Here's the drawing with two shaded views (mm, measured from the low corner). I have some questions. Give positions to 0.01 mm unless a question says otherwise; leave off trailing zeros. Loops run counter-clockwise (first coordinate to the right, second up) from the corner with the lowest first, then second, coordinate; pieces in that order, holes last. Notation, with made-up numbers: (-5.75, -38) - (44.25, -38) arc R29 cw to (44.25, -17) - close; hole circle Ø1 at (31.25, 16.25). An arc over 180 degrees is marked (long way). Answer as a JSON object with one key per item and string values. Group by question number.
Item 1: Suppose I cut it at B-B on z = 24. Write out the boundary of the cut face in (x, y), and give its area (3 significant figures).
Item 2: Suppose I cut it at A-A on x = 24. Write out the boundary of the cut face in (y, z), and give its area (3 significant figures).
Item 3: Suppose I cut it at C-C on y = 1.95. Write out the boundary of the cut face in (x, z), and give its area (3 significant figures).
Item 4: Thinking about a two-plate mould opening in X: for the marked faces 1 and 2, which applies, pulls with the +X half, pulls with the -X half, needs draft (parallel to the pull), parting line crosses it, or undercut?
Item 5: Will these pins go through, and if not, where does the flat tip stop? pin 1 (1.5 mm diameter, centred on x = 35, y = 0.5, fed in from -Z); pin 2 (7 mm diameter, centred on x = 20, z = 27, fed in from -Y).
Item 6: Please list where these lines run through material, in increasing order: L1, parallel to X at y = 0.3, z = 24; L2, parallel to Y at x = 39, z = 29; L3, parallel to X at y = 1.15, z = 26.5.
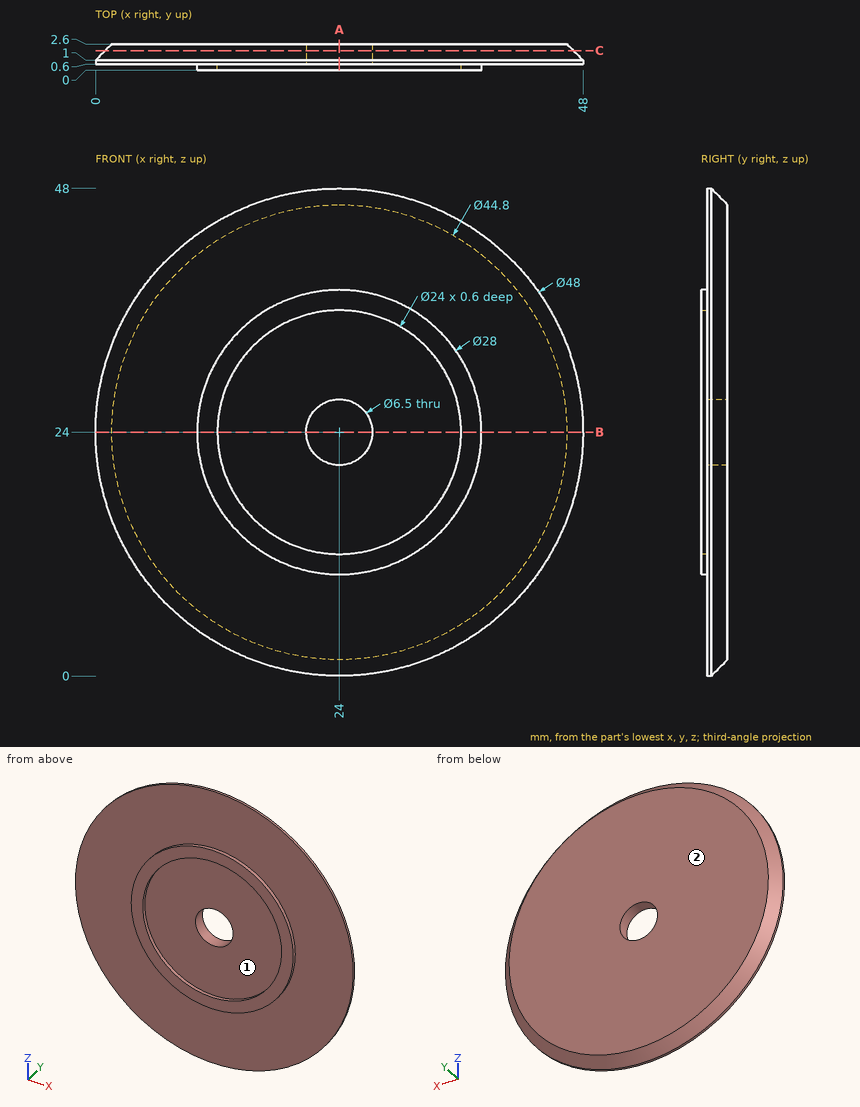
Worked out:
{
 "1": {"outline": "(0, 0.6) - (10, 0.6) - (10, 0) - (12, 0) - (12, 0.6) - (20.75, 0.6) - (20.75, 2.6) - (1.6, 2.6) - (0, 1) - close; (27.25, 0.6) - (36, 0.6) - (36, 0) - (38, 0) - (38, 0.6) - (48, 0.6) - (48, 1) - (46.4, 2.6) - (27.25, 2.6) - close", "area": "82.8 mm2"},
 "2": {"outline": "(0, 10) - (0.6, 10) - (0.6, 0) - (1, 0) - (2.6, 1.6) - (2.6, 20.75) - (0.6, 20.75) - (0.6, 12) - (0, 12) - close; (0, 36) - (0.6, 36) - (0.6, 27.25) - (2.6, 27.25) - (2.6, 46.4) - (1, 48) - (0.6, 48) - (0.6, 38) - (0, 38) - close", "area": "82.8 mm2"},
 "3": {"outline": "circle Ø46.1 at (24, 24); hole circle Ø6.5 at (24, 24)", "area": "1,640 mm2"},
 "4": {"face 1": "undercut", "face 2": "needs draft"},
 "5": {"pin 1": "stops at z = 2.3", "pin 2": "stops at y = 0.6"},
 "6": {"L1": "x = 10 to 12, 36 to 38", "L2": "y = 0.6 to 2.6", "L3": "x = 0.28 to 21.92, 26.08 to 47.72"}
}
